```python
from build123d import *

# Parameters (mm, degrees)
SKETCH_1_W          = 102
SKETCH_1_H          = 100
EXTRUDE_1_DEPTH     = 53
CUT_EXTRUDE_1_DEPTH = 48
SKETCH_3_W          = 51
SKETCH_3_H          = 50
CUT_EXTRUDE_2_DEPTH = 48
CUT_EXTRUDE_3_DEPTH = 48
CHAMFER_1_SIZE      = 15
FILLET_2_R          = 5
SKETCH_5_W          = 100
SKETCH_5_H          = 10
EXTRUDE_2_DEPTH     = 30
SKETCH_6_W          = 10
SKETCH_6_H          = 100
EXTRUDE_3_DEPTH     = 43
FILLET_START        = 5
FILLET_5_DEPTH      = 49
SKETCH_8_R          = 2.5
CUT_EXTRUDE_4_DEPTH = 30
SKETCH_9_R          = 6
CUT_EXTRUDE_5_DEPTH = 7
SKETCH_10_R         = 2.5
CUT_EXTRUDE_6_DEPTH = 30
SKETCH_11_R         = 6
CUT_EXTRUDE_7_DEPTH = 7
CHAMFER_2_SIZE      = 2
FILLET_7_R          = 1


with BuildPart() as part:
    # 草图1 → 凸台-拉伸1 (new body)
    with BuildSketch(Plane(origin=(0, 0, 0), x_dir=(1, 0, 0), z_dir=(0, 1, 0))):
        Rectangle(SKETCH_1_W, SKETCH_1_H)
    extrude(amount=EXTRUDE_1_DEPTH)

    # 草图2 → 切除-拉伸1 (cut)
    with BuildSketch(Plane(origin=(0, 53, 0), x_dir=(1, 0, 0), z_dir=(0, 1, 0))):
        with BuildLine():
            Line((23, -30), (23, 30))
            Line((23, 30), (36.18010503, 30))
            ThreePointArc((36.18010503, 30), (-47, 0), (36.18010503, -30))
            Line((36.18010503, -30), (23, -30))
        make_face()
        with BuildLine():
            Line((36.18010503, 30), (23, 30))
            Line((23, 30), (23, -30))
            Line((23, -30), (36.18010503, -30))
            ThreePointArc((36.18010503, -30), (44.21235651, -15.94576846), (47, 0))
            ThreePointArc((47, 0), (44.21235651, 15.94576846), (36.18010503, 30))
        make_face()
        with BuildLine():
            Line((51, 30), (36.18010503, 30))
            ThreePointArc((36.18010503, 30), (44.21235651, 15.94576846), (47, 0))
            ThreePointArc((47, 0), (44.21235651, -15.94576846), (36.18010503, -30))
            Line((36.18010503, -30), (51, -30))
            Line((51, -30), (51, 30))
        make_face()
    extrude(amount=-CUT_EXTRUDE_1_DEPTH, mode=Mode.SUBTRACT)

    # 草图3 → 切除-拉伸2 (cut)
    with BuildSketch(Plane(origin=(0, 53, 0), x_dir=(1, 0, 0), z_dir=(0, 1, 0))):
        with Locations((25.5, -25)):
            Rectangle(SKETCH_3_W, SKETCH_3_H)
    extrude(amount=-CUT_EXTRUDE_2_DEPTH, mode=Mode.SUBTRACT)

    # 草图4 → 切除-拉伸3 (cut)
    with BuildSketch(Plane(origin=(0, 5, 0), x_dir=(1, 0, 0), z_dir=(0, 1, 0))):
        with BuildLine():
            ThreePointArc((24.5, 22), (22, 24.5), (19.5, 22))
            Line((19.5, 22), (22, 22))
            Line((22, 22), (22, 19.5))
            ThreePointArc((22, 19.5), (23.767766953, 20.232233047), (24.5, 22))
        make_face()
        with BuildLine():
            Line((22, 22), (19.5, 22))
            ThreePointArc((19.5, 22), (20.232233047, 20.232233047), (22, 19.5))
            Line((22, 19.5), (22, 22))
        make_face()
        with BuildLine():
            Line((-22, 19.5), (-22, 22))
            Line((-22, 22), (-19.5, 22))
            ThreePointArc((-19.5, 22), (-23.767766953, 23.767766953), (-22, 19.5))
        make_face()
        with BuildLine():
            Line((-19.5, 22), (-22, 22))
            Line((-22, 22), (-22, 19.5))
            ThreePointArc((-22, 19.5), (-20.232233047, 20.232233047), (-19.5, 22))
        make_face()
        with BuildLine():
            ThreePointArc((-19.5, -22), (-20.232233047, -20.232233047), (-22, -19.5))
            Line((-22, -19.5), (-22, -22))
            Line((-22, -22), (-19.5, -22))
        make_face()
        with BuildLine():
            Line((-22, -22), (-22, -19.5))
            ThreePointArc((-22, -19.5), (-23.767766953, -23.767766953), (-19.5, -22))
            Line((-19.5, -22), (-22, -22))
        make_face()
        with BuildLine():
            ThreePointArc((24.5, -22), (23.767766953, -20.232233047), (22, -19.5))
            Line((22, -19.5), (22, -22))
            Line((22, -22), (19.5, -22))
            ThreePointArc((19.5, -22), (22, -24.5), (24.5, -22))
        make_face()
        with BuildLine():
            Line((22, -22), (22, -19.5))
            ThreePointArc((22, -19.5), (20.232233047, -20.232233047), (19.5, -22))
            Line((19.5, -22), (22, -22))
        make_face()
    extrude(amount=-CUT_EXTRUDE_3_DEPTH, mode=Mode.SUBTRACT)

    # 倒角1
    chamfer_1_edges = [part.edges().sort_by_distance(p)[0] for p in [
        (51, 2.5, 50),
        (51, 26.5, -50),
    ]]
    chamfer(chamfer_1_edges, length=CHAMFER_1_SIZE)

    # 圆角2
    # the kernel refuses this fillet: 5 mm, written as the material it takes off along each edge
    with BuildSketch(Plane(origin=(0, 5, 47), x_dir=(-0.9989898744385596, 0, -0.0449358517136451), z_dir=(0, 1, 0))) as fillet_2_piece_1:
        with BuildLine():
            CenterArc((4.44864932, 4.994949372), FILLET_2_R, 203.55292178, 63.871576317)
            Line((-0.134807555, 2.996969623), (0, 0))
            ThreePointArc((0, 0), (2.111985031, 0.047475901), (4.223970061, 0))
        make_face()
    extrude(amount=58.559925153, mode=Mode.SUBTRACT)
    with BuildSketch(Plane(origin=(36.18010503, 58.69416004, -30), x_dir=(1, 0, 0), z_dir=(0, -1, 0))) as fillet_2_piece_2:
        with BuildLine():
            CenterArc((2.277664016, -5), FILLET_2_R, 90, 47.695010293)
            ThreePointArc((-1.420198392, -1.634615385), (-0.700684154, -0.825487738), (0, 0))
            Line((0, 0), (2.277664016, 0))
        make_face()
    extrude(amount=53.69416004, mode=Mode.SUBTRACT)

    # 草图5 → 凸台-拉伸2 (add)
    with BuildSketch(Plane.ZY.offset(51)):
        with Locations((0, 48)):
            Rectangle(SKETCH_5_W, SKETCH_5_H)
    extrude(amount=EXTRUDE_2_DEPTH)

    # 草图6 → 凸台-拉伸3 (add)
    with BuildSketch(Plane.XZ.offset(-43)):
        with Locations((-76, 0)):
            Rectangle(SKETCH_6_W, SKETCH_6_H)
    extrude(amount=EXTRUDE_3_DEPTH)

    # 圆角5: read off the stored shape, not the designer's step
    # 圆角5 outline → 圆角5 (cut)
    with BuildSketch(Plane(origin=(0, 0, 0), x_dir=(1, 0, 0), z_dir=(0, 1, 0)).offset(FILLET_START)):
        with BuildLine():
            ThreePointArc((-9.446863606, -46.040816327), (-7.859088048, -48.202030509), (-9.848857802, -50))
            Line((-9.848857802, -50), (0, -50))
            ThreePointArc((0, -50), (-1.653487381, -47.801385193), (-4.219703321, -46.810192308))
            ThreePointArc((-4.219703321, -46.810192308), (-6.844103136, -46.499013455), (-9.446863606, -46.040816327))
        make_face()
    extrude(amount=FILLET_5_DEPTH, mode=Mode.SUBTRACT)

    # 草图8 → 切除-拉伸4 (cut)
    with BuildSketch(Plane.XZ.offset(-43)):
        with Locations(Location((-61, 42, 0), (0, 0, 270))):
            Circle(SKETCH_8_R)
        with Locations(Location((-61, -42, 0), (0, 0, 270))):
            Circle(SKETCH_8_R)
    extrude(amount=-CUT_EXTRUDE_4_DEPTH, mode=Mode.SUBTRACT)

    # 草图9 → 切除-拉伸5 (cut)
    with BuildSketch(Plane(origin=(0, 53, 0), x_dir=(1, 0, 0), z_dir=(0, 1, 0))):
        with Locations(Location((-61, 42, 0), (0, 0, 270))):
            Circle(SKETCH_9_R)
        with Locations(Location((-61, -42, 0), (0, 0, 270))):
            Circle(SKETCH_9_R)
    extrude(amount=-CUT_EXTRUDE_5_DEPTH, mode=Mode.SUBTRACT)

    # 草图10 → 切除-拉伸6 (cut)
    with BuildSketch(Plane(origin=(-71, 0, 0), x_dir=(0, 0, -1), z_dir=(1, 0, 0))):
        with Locations((-42, 33)):
            Circle(SKETCH_10_R)
        with Locations((42, 33)):
            Circle(SKETCH_10_R)
    extrude(amount=-CUT_EXTRUDE_6_DEPTH, mode=Mode.SUBTRACT)

    # 草图11 → 切除-拉伸7 (cut)
    with BuildSketch(Plane.ZY.offset(81)):
        with Locations((-42, 33)):
            Circle(SKETCH_11_R)
        with Locations((42, 33)):
            Circle(SKETCH_11_R)
    extrude(amount=-CUT_EXTRUDE_7_DEPTH, mode=Mode.SUBTRACT)

    # 倒角2
    chamfer_2_edges = [part.edges().sort_by_distance(p)[0] for p in [
        (-71, 0, 0),
        (-51, 0, 0),
    ]]
    chamfer(chamfer_2_edges, length=CHAMFER_2_SIZE)

    # 圆角7
    fillet_7_edges = [part.edges().sort_by_distance(p)[0] for p in [
        (-51, 43, 0),
        (-71, 43, 0),
    ]]
    fillet(fillet_7_edges, radius=FILLET_7_R)


solid = part.part
```
Geometry: final body of the model. Coordinates: model frame, mm. A direction names the side the tool comes from. Give positions to 0.01 mm unless a question says otherwise; leave off trailing zeros. Write each loop counter-clockwise with the first axis right and the second up, starting at its lowest first coordinate (ties: lowest second). Pieces come first, ordered by that corner, then holes.
1. Draft query along X for faces 5 (the flat face through (-51, 22, 1)), 6 (the flat face through (-23, 27, -50)), 7 (the flat face through (51, 4.8, -12.8)). Return one class per face: released by +X, released by -X, zero draft, split by the parting line, or undercut.
2. Section query B-B, the plane z = -42. Count the separate pieces of the cut face and the enclosed holes in it, then the cut area to 3 significant figures.
3. Section query A-A, the plane x = -61. Return loops of the section in (y, z), then the cut area to 3 significant figures.
4. Line query: probe 1 along Z at (x, y) = (-22, 3.1); probe 2 along X at (y, z) = (1, 22); probe 3 along X at (y, z) = (1.8, 22). Output: solid intervals per line, ascending.
5. Pin query (flat end, axial travel): P1, Ø14.5, axis at x = -65.5, z = 7.5, coming from the -Y side; P2, Ø1, axis at x = 0, y = 23, coming from the +Z side; P3, Ø3.5, axis at y = 34.5, z = -40, coming from the -X side. Return the tip coordinate at first contact, or that it passes through.
6. Section query C-C, the plane y = 11. Return loops of the section in (x, z), then the cut area to 3 significant figures.
7. Reachability of faces 1 (the cylindrical face through (-61, 50, 36)), 2 (the cylindrical face through (-77.55, 29.35, -46.76)), 3 (the flat face through (45, 29, -30)), 4 (the cylindrical face through (-7.855, 28.664, 48.161)) from +Z, -Z, +X, -X, +Y, -Y: full face, straight path, thin tool, end or side. Return the list, or none.
Computed:
1. face 5: undercut
1. face 6: zero draft
1. face 7: released by +X
2. separate pieces: 3
2. enclosed holes: 0
2. area: 3,540 mm2
3. outline: (43, -50) - (53, -50) - (53, -48) - (46, -48) - (46, -44.5) - (43, -44.5) - close; (43, -39.5) - (46, -39.5) - (46, -36) - (53, -36) - (53, 36) - (46, 36) - (46, 39.5) - (43, 39.5) - close; (43, 44.5) - (46, 44.5) - (46, 48) - (53, 48) - (53, 50) - (43, 50) - close
3. area: 802 mm2
4. probe 1: z = -50 to -24.5, -19.5 to 19.5, 24.5 to 50
4. probe 2: x = -81 to -72, -50 to -24.5, -19.5 to 19.5, 24.5 to 51
4. probe 3: x = -81 to -71.2, -50.8 to -24.5, -19.5 to 19.5, 24.5 to 51
5. P1: stops at y = 0.25
5. P2: stops at z = -47
5. P3: stops at x = -74
6. outline: (-81, -50) - (-71, -50) - (-71, 50) - (-81, 50) - close; (-51, -50) - (36, -50) - (51, -35) - (51, -30) - (38.46, -30) arc R5 ccw to (34.76, -31.63) arc R47 cw (long way) to (-9.45, 46.04) arc R2 ccw to (-9.85, 50) - (-51, 50) - close
6. area: 3,080 mm2
7. face 1: +Y
7. face 2: -X
7. face 3: +Z, +X, +Y
7. face 4: +X, +Y
